Work out the finished part from the listing and answer in its coordinate system (mm). Round coordinates to 2 decimals unless told otherwise and drop trailing zeros. Order: outer loops, then holes, each group sorted by start corner. A loop starts at its lowest first (then second) coordinate and runs counter-clockwise, first axis right, second up. Notation, with made-up numbers: (59.5, 28.5) -> (104.5, 28.5) arc R19 ccw to (104.5, 37.5) -> close; hole circle Ø3 at (2, 1.5). An arc over 180 degrees is marked (long way). Use a Markdown table: item, result. Add a question column.
Item 1: A cutting plane is placed at A-A, the plane y = 0.85. Determine the outline of the cut face in (x, z), plus the area to 3 significant figures.
Item 2: Find the intervals of material crossed by L1, parallel to Z at x = 0, y = 0.95; L2, parallel to Z at x = -0.75, y = 0.2; L3, parallel to X at y = 0.65, z = -1.75, in increasing order. Write a range as [from, to].
Item 3: For a pull along X with two mould halves and no side action, classify faces 1 (the cylindrical face through (1.438, 1.578, 0.748)), 2 (the flat face through (-3, 1.6, -1.8)), 3 (the flat face through (-2, 0, 0)), 4 (the flat face through (3, 1.6, 1.8)) as +X half, -X half, draft (parallel to the pull), parting line (faces both ways), or undercut.
Item 4: Flat-ended cylindrical pins translate along their axes: P1, Ø4, axis at x = 0, z = 0, coming from the -Y side; P2, Ø1, axis at y = 3, z = 2.5, coming from the +X side. Find the tip coordinate at first contact, or state that the pin passes through.
Autodesk Inventor part; units mm, degrees
ref_plane "YZ Plane" through (0, 0, 0) normal (1, 0, 0) x (0, 1, 0)
ref_plane "XZ Plane" through (0, 0, 0) normal (0, 1, 0) x (-1, 0, 0)
ref_plane "XY Plane" through (0, 0, 0) normal (0, 0, 1) x (1, 0, 0)
sketch "スケッチ1" plane through (0, 0, 0) normal (0, 1, 0) x (-1, 0, 0)
  circle A0 centre (0, 0) radius 4.0415 construction
  line L0 (4.0415, 0) -> (2.0207, 3.5)
  line L1 (2.0207, 3.5) -> (-2.0207, 3.5)
  line L2 (-2.0207, 3.5) -> (-4.0415, 0)
  line L3 (-4.0415, 0) -> (-2.0207, -3.5)
  line L4 (-2.0207, -3.5) -> (2.0207, -3.5)
  line L5 (2.0207, -3.5) -> (4.0415, 0)
  dimension "d0" = 7
extrude "押し出し1" add sketch "スケッチ1" along normal blind 3.2
sketch "スケッチ2" plane through (0, 3.2, 0) normal (0, 1, 0) x (1, 0, 0)
  point P0 (0, 0)
  point P1 (0, 0)
hole "穴1" at (0, 3.2, 0) direction (0, -1, 0) diameter 3.242 end through all
sketch "スケッチ3" plane through (0, 0, 0) normal (1, 0, 0) x (0, 1, 0)
  arc A0 (2.4997, -4.5) -> (3.2, -3.5) centre (-2.8622, 0) ccw
  line L0 (0, -3.5) -> (3.2, -3.5) construction
  line L1 (3.2, -4.5) -> (2.4997, -4.5)
  line L2 (3.2, 1.621) -> (3.2, -1.621) construction
  line L3 (3.2, -3.5) -> (3.2, -4.5)
  line L4 (-3.9049, 0) -> (2.5514, 0)
  point P0 (0, 0)
  point P1 (3.2, 0)
  dimension "d10" = 3.5
  dimension "d11" = 7
  dimension "d12" = 1
revolve "回転1" cut sketch "スケッチ3" angle 360 about axis through (0, -10, 0) along (0, 1, 0)
properties part number "M3-HexaNut-type2"
Reported:
| question | item | result |
|---|---|---|
| 1 | outline | (-4.04, 0) -> (-2.02, -3.5) -> (2.02, -3.5) -> (4.04, 0) -> (2.02, 3.5) -> (-2.02, 3.5) -> close; hole circle Ø3.24 at (0, 0) |
| 1 | area | 34.2 mm² |
| 2 | L1 | [-3.5, -1.62], [1.62, 3.5] |
| 2 | L2 | [-3.5, -1.44], [1.44, 3.5] |
| 2 | L3 | [-3.03, 3.03] |
| 3 | face 1 | undercut |
| 3 | face 2 | -X half |
| 3 | face 3 | draft |
| 3 | face 4 | +X half |
| 4 | P1 | y = 0 |
| 4 | P2 | x = 2.89 |
